```python
from build123d import *

# Parameters (mm, degrees)
SKETCH1_W           = 20
SKETCH1_H           = 46
BOSS_EXTRUDE1_DEPTH = 22.86
SKETCH2_R           = 6.05
CUT_EXTRUDE1_DEPTH  = 17.78
FILLET1_R           = 5


with BuildPart() as part:
    # Sketch1 → Boss-Extrude1 (new body)
    with BuildSketch(Plane.XY):
        Rectangle(SKETCH1_W, SKETCH1_H)
    extrude(amount=BOSS_EXTRUDE1_DEPTH)

    # Sketch2 → Cut-Extrude1 (cut)
    with BuildSketch(Plane(origin=(0, 0, 0), x_dir=(-1, 0, 0), z_dir=(0, 0, -1))):
        with Locations((0, 12.5)):
            Circle(SKETCH2_R)
        with Locations((0, -12.5)):
            Circle(SKETCH2_R)
    extrude(amount=-CUT_EXTRUDE1_DEPTH, mode=Mode.SUBTRACT)

    # Fillet1
    fillet1_edges = [part.edges().sort_by_distance(p)[0] for p in [
        (-10, 0, 22.86),
        (0, -23, 22.86),
        (10, 0, 22.86),
        (0, 23, 22.86),
    ]]
    fillet(fillet1_edges, radius=FILLET1_R)


solid = part.part
```
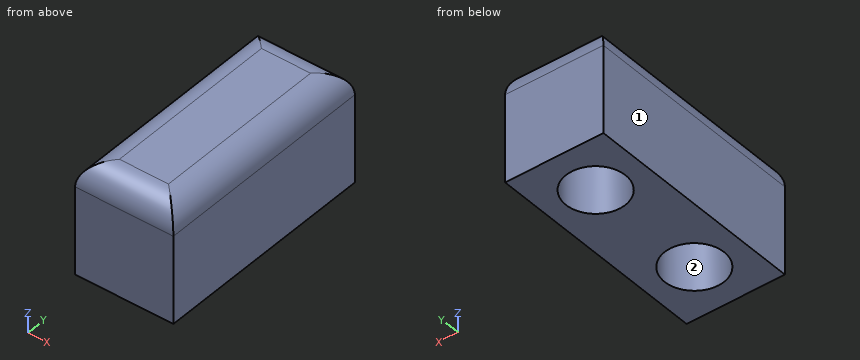
Geometry check sheet. Reference: the model listing, model coordinates, mm. Face numbers are marked on the shaded views. A direction names the side the tool comes from. Coordinates: 2 decimals unless noted, no trailing zeros. Write each loop counter-clockwise with the first axis right and the second up, starting at its lowest first coordinate (ties: lowest second). Pieces come first, ordered by that corner, then holes. Notation, with made-up numbers: M -8,46.5 L -1,46.5 A20 cw -1,72.5 Z; hole C -30,30.25 d3. An arc over 180 degrees is marked long. Use one line per item in the form item = value. Start each with the question number.
1) Section check A-A on y = -12.5. Enter the section's corners in (x, z).
2) Set-up check for the marked faces 1 and 2: record each of +Z, -Z, +X, -X, +Y, -Y from which the full face is reachable in a straight line by a thin tool's end or side.
3) Go/stop test with a flat-tipped pin: pin 1 Ø6 at (x, y) = (2, -13.5) entering from -Z. Record where the tip stops, or that it passes through.
4) Section check D-D on y = 16.5. Enter the section's corners in (x, z).
5) Thickness scan on probe 1 along Y at (x, z) = (0, 7.25); probe 2 along Y at (x, z) = (-3.5, 9.5); probe 3 along X at (y, z) = (-7.5, 3). Record the ranges inside material, lowest first. Write a range as from..to.
6) Section check B-B on x = 0. Enter the section's corners in (y, z).
7) Section check C-C on z = 7.25. Enter the section's corners in (x, y).
Responses:
q1.outline = M -10,0 L -6.05,0 L -6.05,17.78 L 6.05,17.78 L 6.05,0 L 10,0 L 10,17.86 A5 ccw 5,22.86 L -5,22.86 A5 ccw -10,17.86 Z
q2.face_1 = +Z, -Z, -X, +Y, -Y
q2.face_2 = -Z
q3.pin_1 = 17.78
q4.outline = M -10,0 L -4.54,0 L -4.54,17.78 L 4.54,17.78 L 4.54,0 L 10,0 L 10,17.86 A5 ccw 5,22.86 L -5,22.86 A5 ccw -10,17.86 Z
q5.probe_1 = -23..-18.55, -6.45..6.45, 18.55..23
q5.probe_2 = -23..-17.43, -7.57..7.57, 17.43..23
q5.probe_3 = -10..-3.41, 3.41..10
q6.outline = M -23,0 L -18.55,0 L -18.55,17.78 L -6.45,17.78 L -6.45,0 L 6.45,0 L 6.45,17.78 L 18.55,17.78 L 18.55,0 L 23,0 L 23,17.86 A5 ccw 18,22.86 L -18,22.86 A5 ccw -23,17.86 Z
q7.outline = M -10,-23 L 10,-23 L 10,23 L -10,23 Z; hole C 0,-12.5 d12.1; hole C 0,12.5 d12.1
